Source: three-view drawing plus pictorial views. Frame: mm from the lowest corner of the part. A direction names the side the tool comes from. Coordinates: 2 decimals unless noted, no trailing zeros. Write each loop counter-clockwise with the first axis right and the second up, starting at its lowest first coordinate (ties: lowest second). Pieces come first, ordered by that corner, then holes. Notation, with made-up numbers: M 38.5,35 L 64.5,35 A32 ccw 64.5,62 Z; hole C 80.25,83 d7. An arc over 180 degrees is marked long. Use CSV: the item, a comma, the result in double quotes.
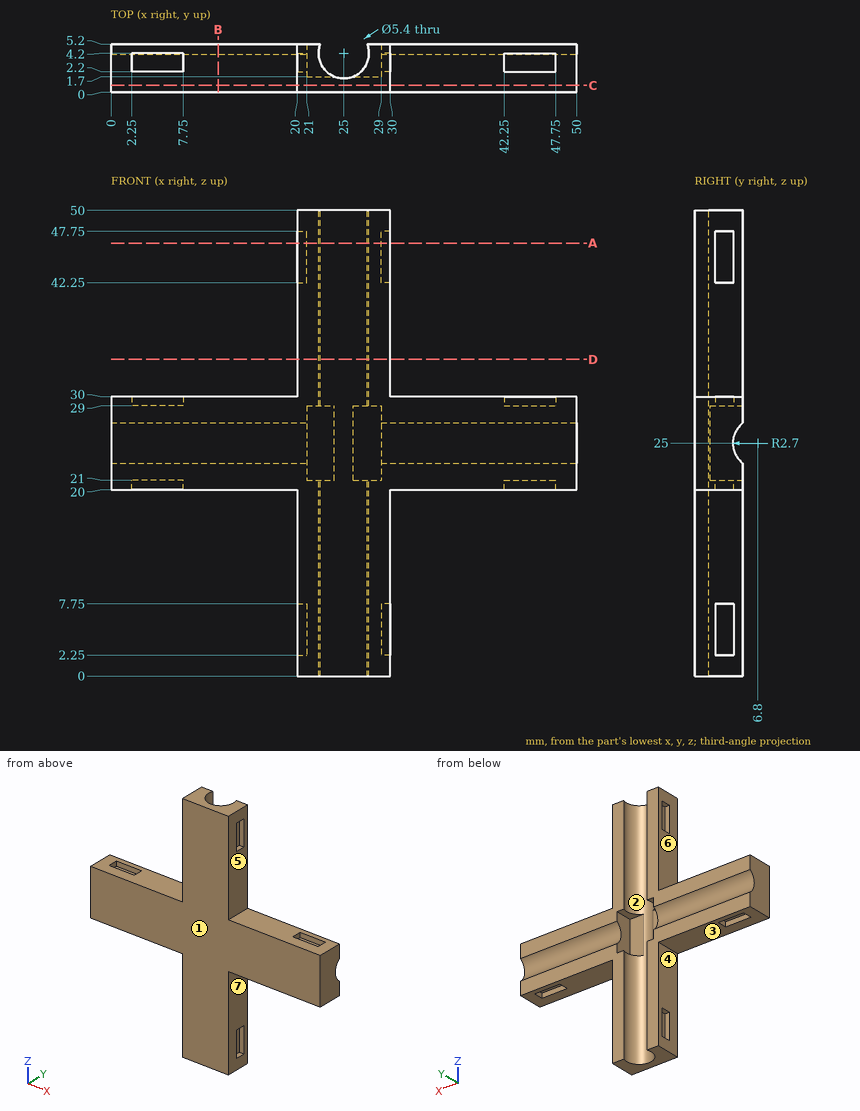
1. Section B-B (x = 11.5). Return loops of the section in (y, z), then the cut area to 3 significant figures.
Resolved:
outline,"M 0,20 L 5.2,20 L 5.2,22.83 A2.7 cw 5.2,27.17 L 5.2,30 L 0,30 Z"
area,"48.7 mm^2"
2. Contact query for flat-ended pins moving along their axis: pin 1 Ø1 at (x, y) = (45.5, 3) entering from +Z; pin 2 Ø1 at (x, y) = (33, 2.5) entering from +Z; pin 3 Ø0.5 at (x, z) = (45.5, 29.5) entering from -Y; pin 4 Ø1.5 at (x, z) = (23, 25) entering from +Y. Output: stop coordinate, or through.
Resolved:
pin 1,"stops at z = 29"
pin 2,"stops at z = 30"
pin 3,"stops at y = 0"
pin 4,"stops at y = 1.7"
3. Section D-D (z = 34). Return loops of the section in (x, y).
Resolved:
outline,"M 20,0 L 30,0 L 30,5.2 L 27.51,5.2 A2.7 cw long 22.49,5.2 L 20,5.2 Z"
4. Access query for the marked faces 4, 5, 6 and 7. Directions: +Z, -Z, +X, -X, +Y, -Y. A direction counts if a zero-diameter tool reaches every point of the face in a straight line with its end or side. Return the directions, or none.
Resolved:
face 4,"-Z, -X, +Y, -Y"
face 5,"+Z, +X, +Y, -Y"
face 6,"+Z, -X, +Y, -Y"
face 7,"-Z, +X, +Y, -Y"
5. Section A-A (z = 46.5). Return loops of the section in (x, y), then the cut area to 3 significant figures.
Resolved:
outline,"M 20,0 L 30,0 L 30,2.2 L 29,2.2 L 29,4.2 L 30,4.2 L 30,5.2 L 27.51,5.2 A2.7 cw long 22.49,5.2 L 20,5.2 L 20,4.2 L 21,4.2 L 21,2.2 L 20,2.2 Z"
area,"31.3 mm^2"
6. Material intervals for line 1 (X direction, y = 4.2, z = 34); line 2 (X direction, y = 4.2, z = 27); line 3 (Z direction, x = 45, y = 1.1), sorted ascending. Write a range as [from, to].
Resolved:
line 1,"x = [20, 22.3], [27.7, 30]"
line 2,"x = [0, 21], [29, 50]"
line 3,"z = [20, 30]"
7. Section C-C (y = 0.75). Return loops of the section in (x, z).
Resolved:
outline,"M 0,20 L 20,20 L 20,0 L 30,0 L 30,20 L 50,20 L 50,30 L 30,30 L 30,50 L 20,50 L 20,30 L 0,30 Z"
8. Mould query, pull axis Y, two halves, no side actions, for the marked faces 1, 2 and 3. Classes: pulls with the +Y half, pulls with the -Y half, needs draft (parallel to the pull), parting line crosses it, or undercut.
Resolved:
face 1,"pulls with the -Y half"
face 2,"undercut"
face 3,"needs draft"
